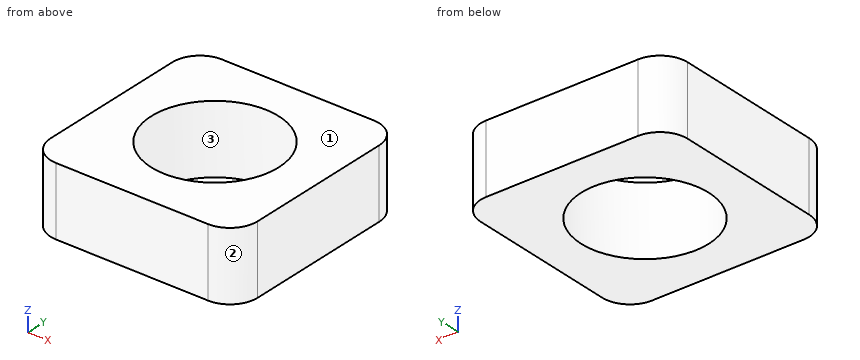
from build123d import *

# Parameters (mm, degrees)
F0_W     = 150
F0_H     = 150
F1_DEPTH = 50
F2_R     = 46.248065
F3_DEPTH = 50
F4_R     = 20
F5_R     = 20
F6_R     = 20


with BuildPart() as f1:
    # F0 (on Top) → F1 (new body)
    with BuildSketch(Plane.XY):
        Rectangle(F0_W, F0_H)
    extrude(amount=F1_DEPTH)

    # F2 (on face) → F3 (cut)
    with BuildSketch(Plane(origin=(0, 0, 0), x_dir=(1, 0, 0), z_dir=(0, 0, -1))):
        Circle(F2_R)
    extrude(amount=-F3_DEPTH, mode=Mode.SUBTRACT)

    # F4
    f4_edges = [f1.edges().sort_by_distance(p)[0] for p in [
        (75, -75, 25),
        (75, 75, 25),
    ]]
    fillet(f4_edges, radius=F4_R)

    # F5
    f5_edges = [f1.edges().sort_by_distance(p)[0] for p in [
        (-75, -75, 25),
    ]]
    fillet(f5_edges, radius=F5_R)

    # F6
    f6_edges = [f1.edges().sort_by_distance(p)[0] for p in [
        (-75, 75, 25),
    ]]
    fillet(f6_edges, radius=F6_R)


solid = f1.part
Can you work these out from the model? Positions are in its coordinate system, mm. Face numbers are marked on the shaded views. Give positions to 0.01 mm unless a question says otherwise; leave off trailing zeros. Order: outer loops, then holes, each group sorted by start corner. A loop starts at its lowest first (then second) coordinate and runs counter-clockwise, first axis right, second up. Notation, with made-up numbers: M -18.5,-8 L 15.5,-8 A27 cw 15.5,25 Z; hole C -23.75,-21 d2. An arc over 180 degrees is marked long. Use a Markdown table: item, result. Add a question column.
Item 1: We'd pull the mould along Y, two halves only. Please class the marked faces 1, 2 and 3: +Y half, -Y half, draft (parallel to the pull), parting line (faces both ways), or undercut.
Item 2: Suppose I cut it at A-A (z = 4.5). List the corners of the cut face in (x, y) for me.
Item 3: Suppose I cut it at B-B (x = 0). List the corners of the cut face in (y, z) for me.
Item 4: If I drill on L1, parallel to Y at x = 0, z = 37; L2, parallel to X at y = -10, z = 5, over which ranges is the centre line in solid material (lowest first)? Write a range as [from, to].
Answer sheet:
| question | item | result |
|---|---|---|
| 1 | face 1 | draft |
| 1 | face 2 | -Y half |
| 1 | face 3 | undercut |
| 2 | outline | M -75,-55 A20 ccw -55,-75 L 55,-75 A20 ccw 75,-55 L 75,55 A20 ccw 55,75 L -55,75 A20 ccw -75,55 Z; hole C 0,0 d92.5 |
| 3 | outline | M -75,0 L -46.25,0 L -46.25,50 L -75,50 Z; M 46.25,0 L 75,0 L 75,50 L 46.25,50 Z |
| 4 | L1 | y = [-75, -46.25], [46.25, 75] |
| 4 | L2 | x = [-75, -45.15], [45.15, 75] |
